Check sheet for the modelled part. Datum: model origin and axes. Units: mm. A direction names the side the tool comes from. Coordinates: 2 decimals unless noted, no trailing zeros. Order: outer loops, then holes, each group sorted by start corner. A loop starts at its lowest first (then second) coordinate and runs counter-clockwise, first axis right, second up.
from build123d import *

# Parameters (mm, degrees)
F0_R      = 38.1
F1_DEPTH  = 101.6
F2_R      = 2.54
F4_R      = 2.54
F6_R      = 12.7
F7_DEPTH  = 50.8
F8_R      = 15.875
F9_DEPTH  = 50.8
F11_R     = 31.75
F12_DEPTH = 2.54


with BuildPart() as f1:
    # F0 (on Top) → F1 (new body)
    with BuildSketch(Plane.XY):
        Circle(F0_R)
    extrude(amount=F1_DEPTH)

    # F2 (on Front) → F3 (revolve, cut)
    with BuildSketch(Plane.XZ):
        with Locations((38.108225, 91.173758)):
            Circle(F2_R)
    revolve(axis=Axis((0, 0, 0), (0, 0, -1)), mode=Mode.SUBTRACT)

    # F4 (on Front) → F5 (revolve, cut)
    with BuildSketch(Plane.XZ):
        with Locations((38.096763, 75.933771)):
            Circle(F4_R)
    revolve(axis=Axis((0, 0, 0), (0, 0, -1)), mode=Mode.SUBTRACT)

    # F6 (on Front) → F7 (cut, symmetric)
    with BuildSketch(Plane.XZ):
        with Locations((0, 31.75)):
            Circle(F6_R)
    extrude(amount=F7_DEPTH, both=True, mode=Mode.SUBTRACT)

    # F8 (on Right) → F9 (cut, symmetric)
    with BuildSketch(Plane.YZ):
        Circle(F8_R)
    extrude(amount=F9_DEPTH, both=True, mode=Mode.SUBTRACT)

    # F11 (on offset) → F12 (cut)
    with BuildSketch(Plane.XY.offset(101.6)):
        Circle(F11_R)
    extrude(amount=-F12_DEPTH, mode=Mode.SUBTRACT)


solid = f1.part
(1) Cross-section at B-B (z = 31.75). Enter the section's corners in (x, y), and give its area (3 significant figures).
Filled in:
outline: (-12.7, -35.92) - (-12.7, 35.92) arc R38.1 ccw to start; (12.7, -35.92) arc R38.1 ccw to (12.7, 35.92) - close
area: 2,660 mm2
(2) Cross-section at A-A (z = 83.5). Enter the section's corners in (x, y), and give its area (3 significant figures).
Filled in:
outline: circle Ø76.2 at (0, 0)
area: 4,560 mm2
(3) Go/stop test with flat-tipped pins: P1, Ø2, axis at y = -16, z = 36.5, coming from the +X side; P2, Ø5, axis at x = -5.5, z = 72.5, coming from the -Y side; P3, Ø5, axis at x = 4.5, y = 4.5, coming from the -Z side. Record where each tip stops, or that it passes through.
Filled in:
P1: stops at x = 35.02
P2: stops at y = -37.98
P3: stops at z = 14.25
(4) Tool access check on faces 1 (the cylindrical face through (-6.883, -30.995, 100.348)), 2 (the cylindrical face through (-30.235, -23.183, 83.483)). Record the directions out of +Z, -Z, +X, -X, +Y, -Y that give a thin tool (end or side, any length) a straight path to the whole face; none if there is none.
Filled in:
face 1: +Z
face 2: +Z, -Z
(5) Release check for a two-part mould opening along Y. For faces 3 (the flat face through (0, 0, 99.06)), 4 (the cylindrical face through (-30.235, -23.183, 97.602)), 5 (the flat face through (0, 25, 0)) record: +Y half, -Y half, draft (parallel to the pull), parting line (faces both ways), or undercut.
Filled in:
face 3: undercut
face 4: parting line
face 5: draft
(6) Thickness scan on probe 1 along X at (y, z) = (0.5, 68.5); probe 2 along Z at (x, y) = (0, -11.5); probe 3 along X at (y, z) = (5.5, 31.75). Record the ranges inside material, lowest first.
Filled in:
probe 1: x = -38.1 to 38.1
probe 2: z = 10.94 to 19.05, 44.45 to 99.06
probe 3: x = -37.7 to -12.7, 12.7 to 37.7
